```python
from build123d import *

# Parameters (mm, degrees)
F0_W     = 44.45
F0_H     = 31.75
F1_DEPTH = 6.35
F2_W     = 9.525
F2_H     = 6.35
F3_DEPTH = 13.97
F5_DEPTH = 31.751
F6_R     = 12.7
F7_R     = 0.508


with BuildPart() as f1:
    # F0 (on Top) → F1 (new body)
    with BuildSketch(Plane.XY):
        Rectangle(F0_W, F0_H)
    extrude(amount=F1_DEPTH)

    # F2 (on Front) → F3 (cut, symmetric)
    with BuildSketch(Plane.XZ):
        with Locations((-6.0325, 3.175)):
            Rectangle(F2_W, F2_H)
        Polygon((-17.1641401403, 8.7758279101), (-20.1476642113, 7.6899139551), (-16.8610756315, -1.3399139551), (-13.8775515605, -0.254), align=None)
        Polygon((1.8125515605, -0.254), (4.7960756315, -1.3399139551), (8.0826642113, 7.6899139551), (5.0991401403, 8.7758279101), align=None)
    extrude(amount=F3_DEPTH, both=True, mode=Mode.SUBTRACT)

    # F4 (on face) → F5 (cut, through all)
    with BuildSketch(Plane.XZ.offset(15.875)):
        Polygon((22.225, 6.35), (10.7699754152, 6.35), (14.5799754152, 2.54), (22.225, 2.54), align=None)
    extrude(amount=-F5_DEPTH, mode=Mode.SUBTRACT)

    # F6
    f6_edges = [f1.edges().sort_by_distance(p)[0] for p in [
        (22.225, -15.875, 1.27),
        (22.225, 15.875, 1.27),
    ]]
    fillet(f6_edges, radius=F6_R)

    # F7
    f7_edges = [f1.edges().sort_by_distance(p)[0] for p in [
        (-16.281211, 0, 6.35),
        (-19.659975, 0, 6.35),
        (-17.348764, 0, 0),
        (-10.795, 0, 6.35),
        (-1.27, 0, 6.35),
        (4.216211, 0, 6.35),
        (-13.97, 0, 0),
        (-10.795, 0, 0),
        (-1.27, 0, 0),
        (1.905, 0, 0),
        (5.283764, 0, 0),
        (7.594975, 0, 6.35),
        (14.579975, 0, 2.54),
        (20.143102, -10.142489, 2.54),
        (18.505256, -12.155256, 0),
        (-22.225, 0, 0),
        (-6.35, 15.875, 6.35),
        (-22.225, 0, 6.35),
        (-6.35, -15.875, 6.35),
        (-22.225, -15.875, 3.175),
        (-22.225, 15.875, 3.175),
        (-6.35, 15.875, 0),
        (18.505256, 12.155256, 0),
        (22.225, 0, 0),
        (-6.35, -15.875, 0),
        (10.148239, 15.859698, 6.35),
        (12.713492, 15.468231, 4.406484),
        (20.143102, 10.142489, 2.54),
        (10.148239, -15.859698, 6.35),
        (22.225, 0, 2.54),
        (12.713492, -15.468231, 4.406484),
    ]]
    fillet(f7_edges, radius=F7_R)


solid = f1.part
```
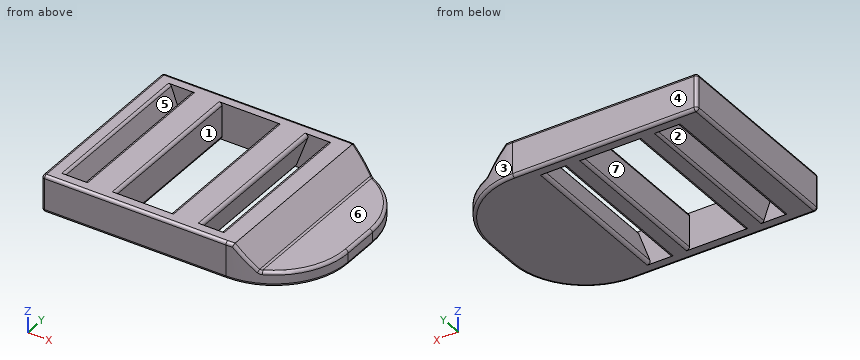
CAD build for the part. Positions are in the model's coordinates, mm. Face numbers are marked on the shaded views. A direction names the side the tool comes from. Give positions to 0.01 mm unless a question says otherwise; leave off trailing zeros. Loops run counter-clockwise (first coordinate to the right, second up) from the corner with the lowest first, then second, coordinate; pieces in that order, holes last. Notation, with made-up numbers: (54.5, -8) - (72.5, -8) arc R30 ccw to (72.5, 27) - close; hole circle Ø11 at (88, -26.75). An arc over 180 degrees is marked (long way). Put each result on its own line as item: value.
Q1. Probe line 1 along Y through (x, z) = (-1.5, 5.5) (3 decimals); line 2 along X through (y, z) = (9, 3.5) (3 decimals); line 3 along X through (y, z) = (13, 0.5). List the from-to ranges inside material, lowest first.
Filled in:
line 1: y = -15.875 to -13.97, 13.97 to 15.875
line 2: x = -22.225 to -18.623, -15.244 to -10.795, -1.27 to 3.179, 6.558 to 13.62
line 3: x = -22.22 to -17.57, -14.15 to -10.8, -1.27 to 2.09, 5.5 to 17.57
Q2. Tool access for the marked faces 5, 6 and 7: list every direction of +Z, -Z, +X, -X, +Y, -Y with a clear straight run to the whole face (end or side of a thin tool).
Filled in:
face 5: +Z
face 6: +Z, +X, +Y, -Y
face 7: +Z, -Z
Q3. Flat gauge pins, fed straight in: pin 1 (10 mm diameter, centred on x = -5, y = -4.5, fed in from -Z); pin 2 (2 mm diameter, centred on x = 19.5, y = 0, fed in from +Z); pin 3 (1.5 mm diameter, centred on y = 6, z = 5, fed in from +X). Where does each tip first touch, or does it go through?
Filled in:
pin 1: stops at z = 0
pin 2: stops at z = 2.54
pin 3: stops at x = 12.87
Q4. Slice it at A-A (z = 1.5). Give the cut face in (x, y) (3 decimals).
Filled in:
outline: (-22.225, -15.367) arc R0.508 ccw to (-21.717, -15.875) - (9.525, -15.875) arc R12.7 ccw to (22.225, -3.175) - (22.225, 3.175) arc R12.7 ccw to (9.525, 15.875) - (-21.717, 15.875) arc R0.508 ccw to (-22.225, 15.367) - close; hole (-17.895, -13.97) - (-14.516, -13.97) - (-14.516, 13.97) - (-17.895, 13.97) - close; hole (-10.795, -13.97) - (-1.27, -13.97) - (-1.27, 13.97) - (-10.795, 13.97) - close; hole (2.451, -13.97) - (5.83, -13.97) - (5.83, 13.97) - (2.451, 13.97) - close
Q5. Slice it at B-B (y = -0.5). Give the number of separate pieces and of enclosed holes in the cut face, plus the area to 3 significant figures.
Filled in:
separate pieces: 4
enclosed holes: 0
area: 141 mm²
Q6. Mould opens along X. For the marked faces 1, 2, 3 and 4 say: pulls with the +X half, pulls with the -X half, needs draft (parallel to the pull), parting line crosses it, or undercut.
Filled in:
face 1: undercut
face 2: undercut
face 3: pulls with the +X half
face 4: needs draft
